For this review, take the finished solid that the model builds, in its own axes (mm). A direction names the side the tool comes from. Coordinates: 2 decimals unless noted, no trailing zeros. Loops run counter-clockwise (first coordinate to the right, second up) from the corner with the lowest first, then second, coordinate; pieces in that order, holes last. Notation, with made-up numbers: (-20.75, 3) -> (38.25, 3) arc R25 ccw to (38.25, 15) -> close; hole circle Ø10 at (-2.75, 8.25). An arc over 180 degrees is marked (long way). One line per item, written item: value.
from build123d import *

# Parameters (mm, degrees)
BOSS_EXTRUDE1_DEPTH   = 14.90345
F_8_CLEARANCE_HOLE1_D = 4.4958
CUT_EXTRUDE1_START    = -13.084175
CUT_EXTRUDE1_DEPTH    = 13.084175
F_6_CLEARANCE_HOLE1_D = 3.7973


with BuildPart() as part:
    # Sketch1 → Boss-Extrude1 (new body)
    with BuildSketch(Plane(origin=(0, 0, 0), x_dir=(0, 0, -1), z_dir=(1, 0, 0))):
        with BuildLine():
            Line((-12.390427979, -33.883508061), (14.444672021, -16.268608061))
            ThreePointArc((14.444672021, -16.268608061), (14.622989145, -16.14717462), (14.797078303, -16.019753892))
            Line((14.797078303, -16.019753892), (29.249678303, -5.059653892))
            ThreePointArc((29.249678303, -5.059653892), (31.7627, 0), (29.249678303, 5.059653892))
            Line((29.249678303, 5.059653892), (14.797078303, 16.019753892))
            ThreePointArc((14.797078303, 16.019753892), (14.622989145, 16.14717462), (14.444672021, 16.268608061))
            Line((14.444672021, 16.268608061), (-12.390427979, 33.883508061))
            ThreePointArc((-12.390427979, 33.883508061), (-20.503514332, 32.92233885), (-20.955, 24.765))
            ThreePointArc((-20.955, 24.765), (-18.474577219, 21.05577373), (-16.409060049, 17.100461415))
            ThreePointArc((-16.409060049, 17.100461415), (-15.641722595, 14.450337743), (-15.666107705, 11.691467029))
            ThreePointArc((-15.666107705, 11.691467029), (-15.575146808, 9.784196429), (-14.742333624, 8.065948127))
            ThreePointArc((-14.742333624, 8.065948127), (-13.400723388, 5.655129962), (-12.806341132, 2.960937694))
            ThreePointArc((-12.806341132, 2.960937694), (-12.7, 0), (-12.806341132, -2.960937694))
            ThreePointArc((-12.806341132, -2.960937694), (-13.400723388, -5.655129962), (-14.742333624, -8.065948127))
            ThreePointArc((-14.742333624, -8.065948127), (-15.575146808, -9.784196429), (-15.666107705, -11.691467029))
            ThreePointArc((-15.666107705, -11.691467029), (-15.641722595, -14.450337743), (-16.409060049, -17.100461415))
            ThreePointArc((-16.409060049, -17.100461415), (-18.474577219, -21.05577373), (-20.955, -24.765))
            ThreePointArc((-20.955, -24.765), (-20.503514332, -32.92233885), (-12.390427979, -33.883508061))
        make_face()
    extrude(amount=BOSS_EXTRUDE1_DEPTH)

    # #8 Clearance Hole1 (through all)
    with Locations(Plane(origin=(14.90345, 0, 0), x_dir=(0, 0, -1), z_dir=(1, 0, 0))):
        with Locations((-15.875, -28.575), (-15.875, 28.575), (25.4127, 0)):
            Hole(F_8_CLEARANCE_HOLE1_D / 2)

    # Sketch4 → Cut-Extrude1 (cut)
    with BuildSketch(Plane(origin=(14.90345, 0, 0), x_dir=(0, 0, -1), z_dir=(1, 0, 0)).offset(CUT_EXTRUDE1_START)):
        with BuildLine():
            Line((2.952066637, -17.4625), (-14.703535363, -17.4625))
            ThreePointArc((-14.703535363, -17.4625), (-17.670883965, -16.233383965), (-18.9, -13.266035363))
            Line((-18.9, -13.266035363), (-18.9, 16.569743879))
            Line((-18.9, 16.569743879), (-11.384871939, 24.084871939))
            ThreePointArc((-11.384871939, 24.084871939), (-10.008364969, 26.144960204), (-9.525, 28.575))
            Line((-9.525, 28.575), (-9.525, 39.085699772))
            Line((-9.525, 39.085699772), (17.4625, 39.085699772))
            Line((17.4625, 39.085699772), (17.4625, 20.906374998))
            Line((17.4625, 20.906374998), (22.410286301, 14.224662488))
            ThreePointArc((22.410286301, 14.224662488), (19.145516673, 14.39328975), (17.4625, 11.590681902))
            Line((17.4625, 11.590681902), (17.4625, -17.4625))
            Line((17.4625, -17.4625), (7.616513377, -28.12126277))
            ThreePointArc((7.616513377, -28.12126277), (8.769417563, -21.266733278), (2.952066637, -17.4625))
        make_face()
    extrude(amount=CUT_EXTRUDE1_DEPTH, mode=Mode.SUBTRACT)

    # #6 Clearance Hole1 (through all)
    with Locations(Plane.ZY):
        with Locations((10.9601, -10.9601), (-10.9601, -10.9601), (-10.9601, 10.9601), (10.9601, 10.9601)):
            Hole(F_6_CLEARANCE_HOLE1_D / 2)


solid = part.part
1. For faces 1 (the flat face through (8, 30, 9.525)), 2 (the flat face through (8.27, 21.22, 14.25)), 3 (the cylindrical face through (0.897, 5.691, 13.415)), list the 3-axis set-ups (+Z, -Z, +X, -X, +Y, -Y) from which the entire face can be reached by the end or side of a thin tool; tool diameter is ignored.
Return value:
face 1: -Z, +X, +Y
face 2: -Z, +X
face 3: +Z, +X, -X
2. Take a section at A-A, the plane y = 0. Give the boundary of the cut face in (x, z), and give its area (3 significant figures).
Return value:
outline: (0, -31.76) -> (14.9, -31.76) -> (14.9, -27.66) -> (0, -27.66) -> close; (0, -23.16) -> (14.9, -23.16) -> (14.9, -17.46) -> (1.82, -17.46) -> (1.82, 12.7) -> (0, 12.7) -> close
area: 201 mm2
3. Take a section at C-C, the plane z = -24.5. Give the boundary of the cut face in (x, y).
Return value:
outline: (0, -8.66) -> (14.9, -8.66) -> (14.9, -2.05) -> (0, -2.05) -> close; (0, 2.05) -> (14.9, 2.05) -> (14.9, 8.66) -> (0, 8.66) -> close
4. To check wall thickness, follow probe 1 along Y at (x, z) = (11, 15); probe 2 along Y at (x, z) = (11.25, 17.5); probe 3 along X at (y, z) = (-5, 8.5). State the ranges of each line that lie inside material, in increasing order. Write a range as from..to.
Return value:
probe 1: y = -34.86..-30.65, -26.5..-17.45, 20.47..26.5, 30.65..34.86
probe 2: y = -34.71..-30.13, -27.02..-19.32, 19.32..27.02, 30.13..34.71
probe 3: x = 0..1.82
5. Take a section at D-D, the plane z = -11. Give the boundary of the cut face in (x, y), and give its area (3 significant figures).
Return value:
outline: (0, -18.53) -> (1.82, -18.53) -> (1.82, -12.86) -> (0, -12.86) -> close; (0, -9.06) -> (1.82, -9.06) -> (1.82, 9.06) -> (0, 9.06) -> close; (0, 12.86) -> (1.82, 12.86) -> (1.82, 18.53) -> (0, 18.53) -> close
area: 53.6 mm2
6. The part is to be moulded in two halves that separate along Y. For faces 4 (the cylindrical face through (8.27, 12.616, -17.633)), 5 (the flat face through (14.903, 30.5, 17.4)), 6 (the cylindrical face through (0.922, 9.805, 12.467)), say which applies: pulls with the +Y half, pulls with the -Y half, needs draft (parallel to the pull), parting line crosses it, or undercut.
Return value:
face 4: pulls with the +Y half
face 5: needs draft
face 6: undercut
7. Insertion check: pin 1 Ø4 at (x, y) = (6, 30.5) entering from -Z (3 decimals); pin 2 Ø5 at (y, z) = (-10.96, 10.96) entering from -X; pin 3 Ø4 at (x, z) = (11, 1) entering from -Y; pin 4 Ø10.5 at (y, z) = (2.5, 2.5) entering from +X. Each pin has a flat end and moves straight along its axis. Give the tip position at first contact, or say it passes through.
Return value:
pin 1: stops at z = 9.525
pin 2: stops at x = 0
pin 3: stops at y = -27.72
pin 4: stops at x = 1.82
8. Take a section at B-B, the plane x = 13. Give the number of separate pieces and of enclosed holes in the cut face, and give its area (3 significant figures).
Return value:
separate pieces: 3
enclosed holes: 3
area: 665 mm2
